For this review, use the dimensioned drawing (mm, ordinates from the lowest corner) and the shaded views. Coordinates: 2 decimals unless noted, no trailing zeros. Loops run counter-clockwise (first coordinate to the right, second up) from the corner with the lowest first, then second, coordinate; pieces in that order, holes last. Notation, with made-up numbers: M 40.5,80 L 57.5,80 A22 cw 57.5,102 Z; hole C -28,-25 d5. An arc over 180 degrees is marked long. One line per item, written item: value.
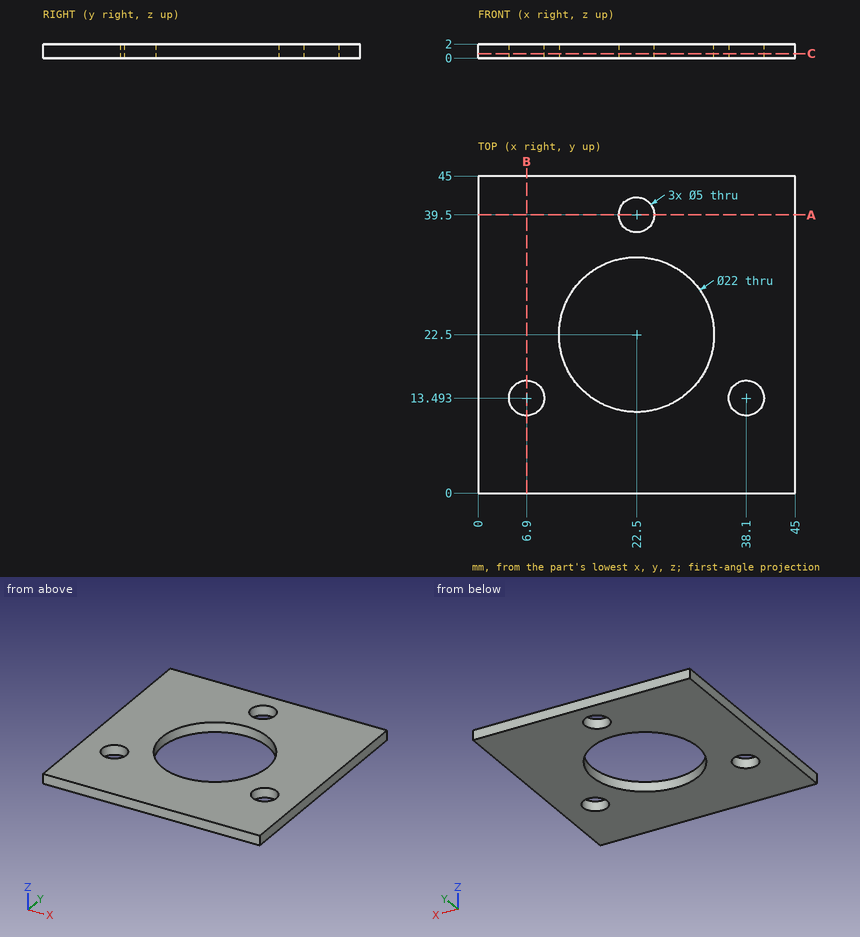
(1) Insertion check: pin 1 Ø20 at (x, y) = (22.5, 22.5) entering from -Z. The pin has a flat end and moves straight along its axis. Give the tip position at first contact, or say it passes through.
Checks:
pin 1: through
(2) Add section C-C on z = 0.65. State the section outline as (x, y) points, then the cut area to 3 significant figures.
Checks:
outline: M 0,0 L 45,0 L 45,45 L 0,45 Z; hole C 6.9,13.49 d5; hole C 22.5,22.5 d22; hole C 22.5,39.5 d5; hole C 38.1,13.49 d5
area: 1,590 mm^2
(3) Add section B-B on x = 6.9. State the section outline as (y, z) points.
Checks:
outline: M 0,0 L 10.99,0 L 10.99,2 L 0,2 Z; M 15.99,0 L 45,0 L 45,2 L 15.99,2 Z
(4) To check wall thickness, follow L1, parallel to Y at x = 22.5, z = 0.55; L2, parallel to X at y = 15, z = 0.85 (1 decimal); L3, parallel to X at y = 23, z = 1.85. State the ranges of each line that lie inside material, in increasing order. Write a range as [from, to].
Checks:
L1: [0, 11.5], [33.5, 37], [42, 45]
L2: [0, 4.9], [8.9, 14.5], [30.5, 36.1], [40.1, 45]
L3: [0, 11.51], [33.49, 45]
(5) Add section A-A on y = 39.5. State the section outline as (x, z) points.
Checks:
outline: M 0,0 L 20,0 L 20,2 L 0,2 Z; M 25,0 L 45,0 L 45,2 L 25,2 Z
